Verification items for the finished model (mm, model axes). Face numbers are marked on the shaded views. A direction names the side the tool comes from. Round coordinates to 2 decimals unless told otherwise and drop trailing zeros. Write each loop counter-clockwise with the first axis right and the second up, starting at its lowest first coordinate (ties: lowest second). Pieces come first, ordered by that corner, then holes. Notation, with made-up numbers: M -1.75,-10 L 15.25,-10 A8 ccw 15.25,5 Z; hole C -17,60 d6. An arc over 180 degrees is marked long. Use a Markdown table: item, result. Add a question column.
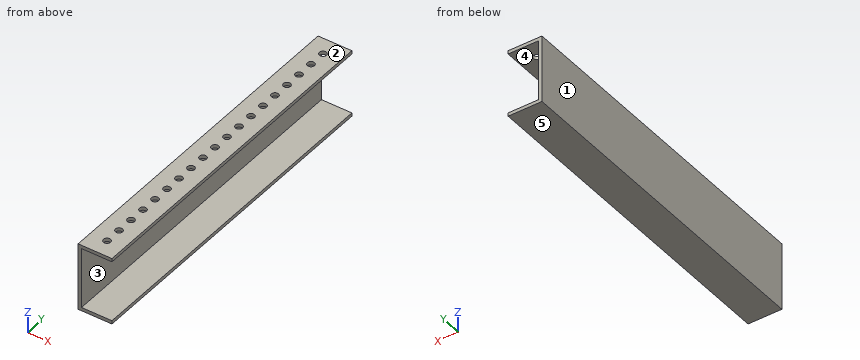
from build123d import *

# Parameters (mm, degrees)
F1_DEPTH = 127
F2_R     = 2.667
F3_DEPTH = 2.54


with BuildPart() as f1:
    # F0 (on Front) → F1 (new body, symmetric)
    with BuildSketch(Plane.XZ):
        Polygon((25.4, 22.86), (25.4, 25.4), (0, 25.4), (0, -25.4), (25.4, -25.4), (25.4, -22.86), (2.54, -22.86), (2.54, 22.86), align=None)
    extrude(amount=F1_DEPTH, both=True)

    # F2 (on face) → F3 (cut)
    with BuildSketch(Plane.XY.offset(25.4)):
        with Locations((12.7, -50.8)):
            Circle(F2_R)
        with Locations((12.7, -63.5)):
            Circle(F2_R)
        with Locations((12.7, -114.3)):
            Circle(F2_R)
        with Locations((12.7, 101.6)):
            Circle(F2_R)
        with Locations((12.7, -76.2)):
            Circle(F2_R)
        with Locations((12.7, 76.2)):
            Circle(F2_R)
        with Locations((12.7, 88.9)):
            Circle(F2_R)
        with Locations((12.7, 50.8)):
            Circle(F2_R)
        with Locations((12.7, -101.6)):
            Circle(F2_R)
        with Locations((12.7, -25.4)):
            Circle(F2_R)
        with Locations((12.7, -38.1)):
            Circle(F2_R)
        with Locations((12.7, 12.7)):
            Circle(F2_R)
        with Locations((12.7, -88.9)):
            Circle(F2_R)
        with Locations((12.7, -12.7)):
            Circle(F2_R)
        with Locations((12.7, 25.4)):
            Circle(F2_R)
        with Locations((12.7, 38.1)):
            Circle(F2_R)
        with Locations((12.7, 0)):
            Circle(F2_R)
        with Locations((12.7, 63.5)):
            Circle(F2_R)
        with Locations((12.7, 114.3)):
            Circle(F2_R)
    extrude(amount=-F3_DEPTH, mode=Mode.SUBTRACT)


solid = f1.part
1. Cross-section at C-C on z = 18. Enter the section's corners in (x, y).
2. Depth check by flat-ended pin: pin 1 Ø10 at (x, z) = (20.5, -15) entering from -Y; pin 2 Ø3 at (x, y) = (12.7, 0) entering from +Z; pin 3 Ø23 at (y, z) = (0.5, -11) entering from +X. Enter the tip coordinate at first touch or a pass-through.
3. Access from +Z, -Z, +X, -X, +Y, -Y to the whole of each face (thin tool, end or side, straight path). Record for the marked faces 4 and 5.
4. Cross-section at A-A on y = 25.4. Enter the section's corners in (x, z).
5. Scan lines: line 1 along Z through (x, y) = (8.5, -13.5); line 2 along X through (y, z) = (-63, 24); line 3 along X through (y, z) = (-69.5, 20). Record each from-to range of solid material in increasing order. Write a range as from..to.
6. Release check for a two-part mould opening along Z. For the marked faces 1, 2 and 3 record: +Z half, -Z half, draft (parallel to the pull), parting line (faces both ways), or undercut.
7. Cross-section at B-B on x = 5.5. Enter the section's corners in (y, z), plus the area to 3 significant figures.
Answer:
| question | item | result |
|---|---|---|
| 1 | outline | M 0,-127 L 2.54,-127 L 2.54,127 L 0,127 Z |
| 2 | pin 1 | passes through |
| 2 | pin 2 | stops at z = -22.86 |
| 2 | pin 3 | stops at x = 2.54 |
| 3 | face 4 | +X, +Y, -Y |
| 3 | face 5 | -Z, +X, -X, +Y, -Y |
| 4 | outline | M 0,-25.4 L 25.4,-25.4 L 25.4,-22.86 L 2.54,-22.86 L 2.54,22.86 L 10.03,22.86 L 10.03,25.4 L 0,25.4 Z; M 15.37,22.86 L 25.4,22.86 L 25.4,25.4 L 15.37,25.4 Z |
| 5 | line 1 | z = -25.4..-22.86, 22.86..25.4 |
| 5 | line 2 | x = 0..10.08, 15.32..25.4 |
| 5 | line 3 | x = 0..2.54 |
| 6 | face 1 | draft |
| 6 | face 2 | +Z half |
| 6 | face 3 | undercut |
| 7 | outline | M -127,-25.4 L 127,-25.4 L 127,-22.86 L -127,-22.86 Z; M -127,22.86 L 127,22.86 L 127,25.4 L -127,25.4 Z |
| 7 | area | 1,290 mm^2 |
